Here's the drawing with two shaded views (mm, measured from the low corner). I have some questions. A direction names the side the tool comes from. Round coordinates to 2 decimals unless told otherwise and drop trailing zeros. Loops run counter-clockwise (first coordinate to the right, second up) from the corner with the lowest first, then second, coordinate; pieces in that order, holes last. Notation, with made-up numbers: (66, 45.25) -> (124, 45.25) arc R21 cw to (124, 82.25) -> close; hole circle Ø7 at (-31.75, 42). An arc over 180 degrees is marked (long way). Write item = value, one per line.
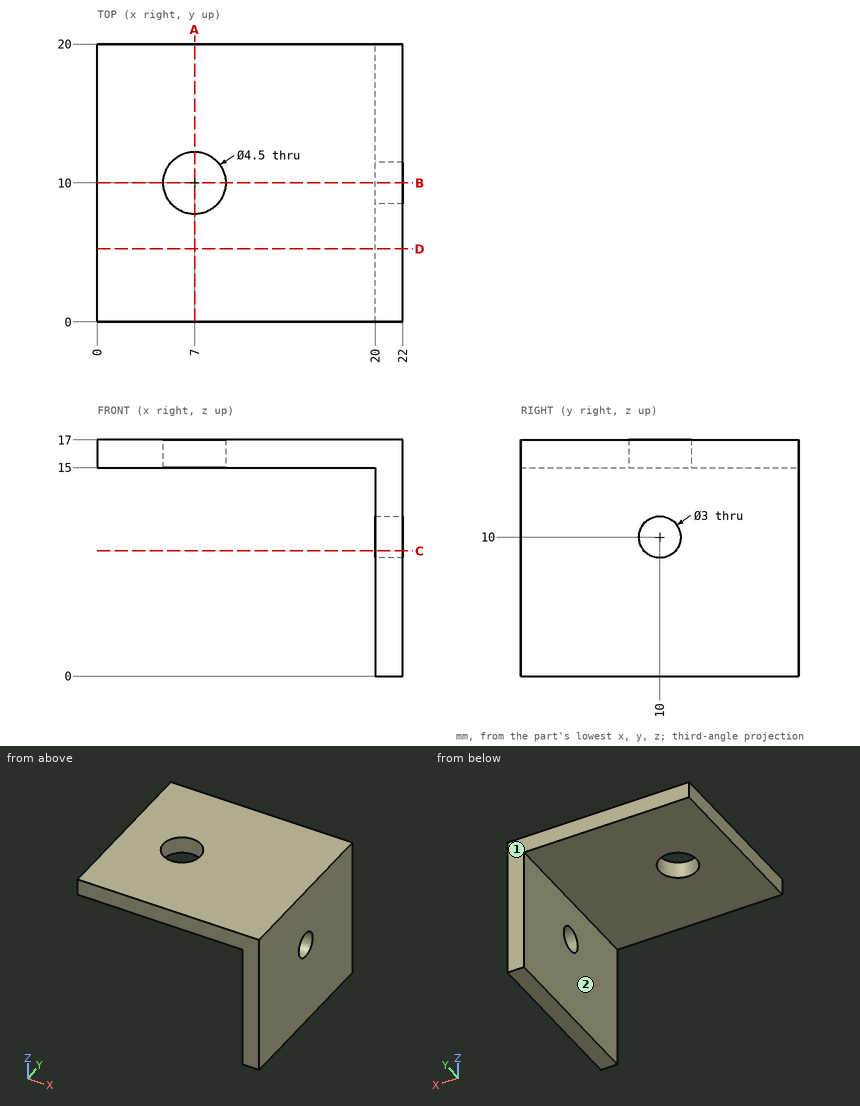
1. For the marked faces 1 and 2, which set-ups out of +Z, -Z, +X, -X, +Y, -Y let a thin tool reach every point of the face, with its end or its side?
Entries:
face_1 = +Z, -Z, +X, -X, +Y
face_2 = -Z, -X, +Y, -Y
2. Suppose I cut it at B-B, the plane y = 10. List the corners of the cut face in (x, z) for me.
Entries:
outline = (0, 15) -> (4.75, 15) -> (4.75, 17) -> (0, 17) -> close; (9.25, 15) -> (20, 15) -> (20, 11.5) -> (22, 11.5) -> (22, 17) -> (9.25, 17) -> close; (20, 0) -> (22, 0) -> (22, 8.5) -> (20, 8.5) -> close
3. I need wall thicknesses on line 1 (Y direction, x = 7, z = 15.4); line 2 (Y direction, x = 21.45, z = 10); line 3 (Z direction, x = 12.5, y = 15.5). Which ranges of each line are inside material? Lowest first, please. Write a range as [from, to].
Entries:
line_1 = [0, 7.75], [12.25, 20]
line_2 = [0, 8.5], [11.5, 20]
line_3 = [15, 17]
4. Suppose I cut it at C-C, the plane z = 9. List the corners of the cut face in (x, y) for me, and give its area (3 significant figures).
Entries:
outline = (20, 0) -> (22, 0) -> (22, 8.88) -> (20, 8.88) -> close; (20, 11.12) -> (22, 11.12) -> (22, 20) -> (20, 20) -> close
area = 35.5 mm²
5. Suppose I cut it at D-D, the plane y = 5.25. List the corners of the cut face in (x, z) for me, and give its area (3 significant figures).
Entries:
outline = (0, 15) -> (20, 15) -> (20, 0) -> (22, 0) -> (22, 17) -> (0, 17) -> close
area = 74.0 mm²
6. I'm going to push flat-ended pins straight in: pin 1 (4.5 mm diameter, centred on y = 11, z = 5, fed in from -X); pin 2 (7 mm diameter, centred on x = 7, y = 10, fed in from -Z). Where does each tip first touch, or does it pass through?
Entries:
pin_1 = 20
pin_2 = 15
7. Suppose I cut it at A-A, the plane x = 7. List the corners of the cut face in (y, z) for me.
Entries:
outline = (0, 15) -> (7.75, 15) -> (7.75, 17) -> (0, 17) -> close; (12.25, 15) -> (20, 15) -> (20, 17) -> (12.25, 17) -> close
